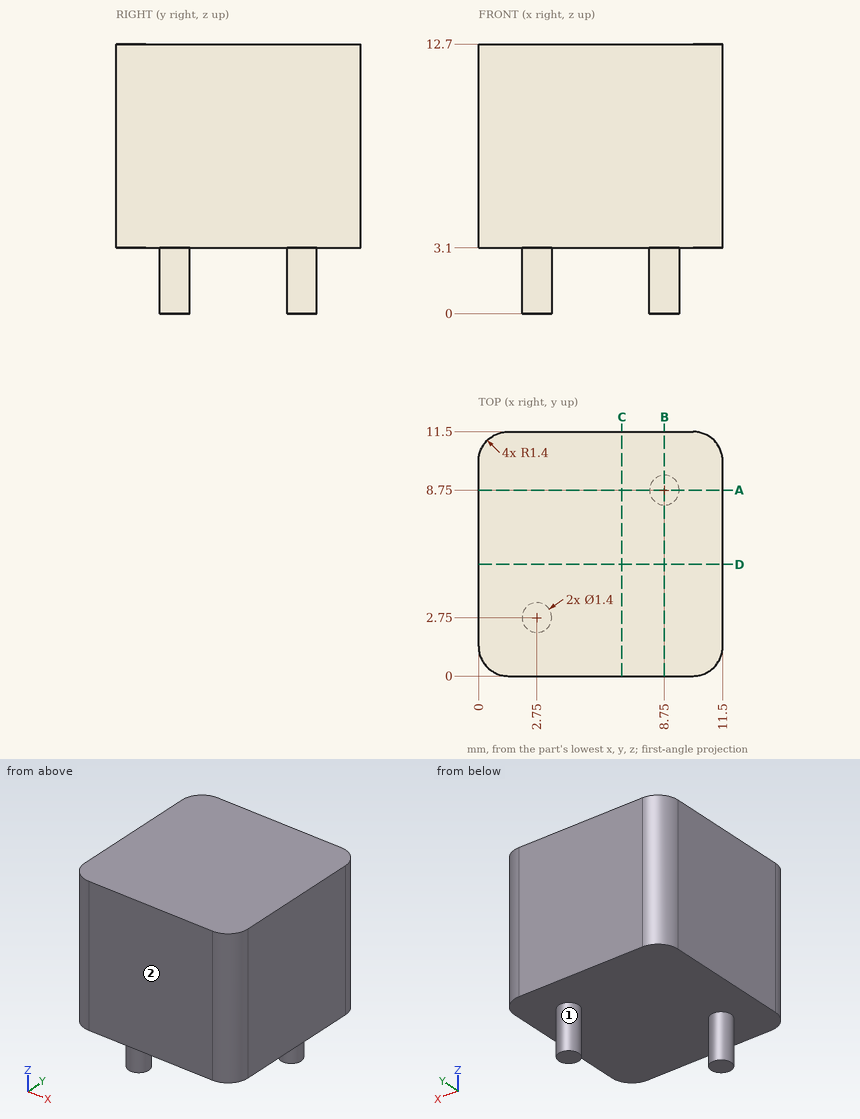
Geometry check sheet. Reference: drawing and pictorial views, mm from the part's lowest x, y, z. A direction names the side the tool comes from. Coordinates: 2 decimals unless noted, no trailing zeros. Write each loop counter-clockwise with the first axis right and the second up, starting at its lowest first coordinate (ties: lowest second). Pieces come first, ordered by that corner, then holes. Notation, with made-up numbers: M 14,-36.5 L 66,-36.5 A35 ccw 66,-2.5 Z; hole C 29,57.25 d2. An arc over 180 degrees is marked long. One line per question, with ' | ' between items.
1) Sectioned sample at A-A on y = 8.75. Record the cut outline in (x, z).
Solutions:
outline: M 0,3.1 L 8.05,3.1 L 8.05,0 L 9.45,0 L 9.45,3.1 L 11.5,3.1 L 11.5,12.7 L 0,12.7 Z
2) Depth check by flat-ended pin: pin 1 Ø6 at (x, y) = (8, 4.5) entering from -Z. Enter the tip coordinate at first touch or a pass-through.
Solutions:
pin 1: z = 3.1
3) Sectioned sample at C-C on x = 6.75. Record the cut outline in (y, z).
Solutions:
outline: M 0,3.1 L 11.5,3.1 L 11.5,12.7 L 0,12.7 Z
4) Access from +Z, -Z, +X, -X, +Y, -Y to the whole of each face (thin tool, end or side, straight path). Record for the marked faces 1 and 2.
Solutions:
face 1: -Z | face 2: +Z, -Z, +X, -X, -Y
5) Material ranges on L1, parallel to Z at x = 9, y = 2; L2, parallel to X at y = 3.25, z = 2.75; L3, parallel to X at y = 10.5, z = 8.75, recorded low to high.
Solutions:
L1: 3.1 to 12.7 | L2: 2.26 to 3.24 | L3: 0.06 to 11.44
